Answer from the drawing. Dimensions are ordinates in mm from the lowest x, y and z of the part. Give positions to 0.01 mm unless a question says otherwise; leave off trailing zeros. Loops run counter-clockwise (first coordinate to the right, second up) from the corner with the lowest first, then second, coordinate; pieces in that order, holes last. Notation, with made-up numbers: (78, 79.25) - (89, 79.25) arc R27 cw to (89, 112.25) - close; hole circle Ø5 at (76.5, -18.75). An arc over 180 degrees is marked (long way). Put each result on its own line as item: value. Start each with the question number.
1. Consider L1, parallel to X at y = 1.55, z = 6.35 (3 decimals); L2, parallel to X at y = 0.3, z = 54 (3 decimals). Determine where each line is inside the solid, lowest interval first. Write a range as from..to.
2. A cutting plane is placed at A-A, the plane y = 1.45. Determine the outline of the cut face in (x, z) (3 decimals).
3. Given pin 1 Ø1.2 at (y, z) = (3, 59.5) entering from +X; pin 2 Ø0.9 at (x, y) = (23.5, 2) entering from +Z; pin 3 Ø0.9 at (x, y) = (148.5, 2) entering from -Z, each flat-ended and moving along its own axis, determine where each tip first touches the part or whether it passes through.
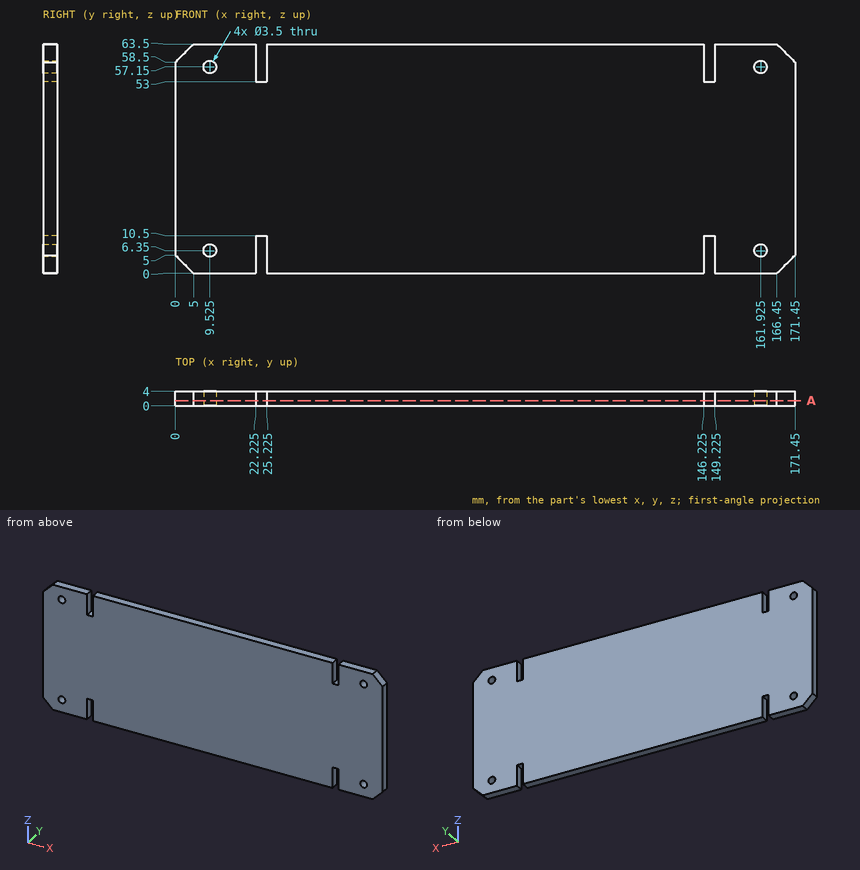
Return value:
1. L1: x = 0..7.775, 11.275..22.225, 25.225..146.225, 149.225..160.175, 163.675..171.45
1. L2: x = 0..22.225, 25.225..146.225, 149.225..171.45
2. outline: (0, 5) - (5, 0) - (22.225, 0) - (22.225, 10.5) - (25.225, 10.5) - (25.225, 0) - (146.225, 0) - (146.225, 10.5) - (149.225, 10.5) - (149.225, 0) - (166.45, 0) - (171.45, 5) - (171.45, 58.5) - (166.45, 63.5) - (149.225, 63.5) - (149.225, 53) - (146.225, 53) - (146.225, 63.5) - (25.225, 63.5) - (25.225, 53) - (22.225, 53) - (22.225, 63.5) - (5, 63.5) - (0, 58.5) - close; hole circle Ø3.5 at (9.525, 6.35); hole circle Ø3.5 at (9.525, 57.15); hole circle Ø3.5 at (161.925, 6.35); hole circle Ø3.5 at (161.925, 57.15)
3. pin 1: stops at x = 171.05
3. pin 2: stops at z = 53
3. pin 3: stops at z = 10.5
